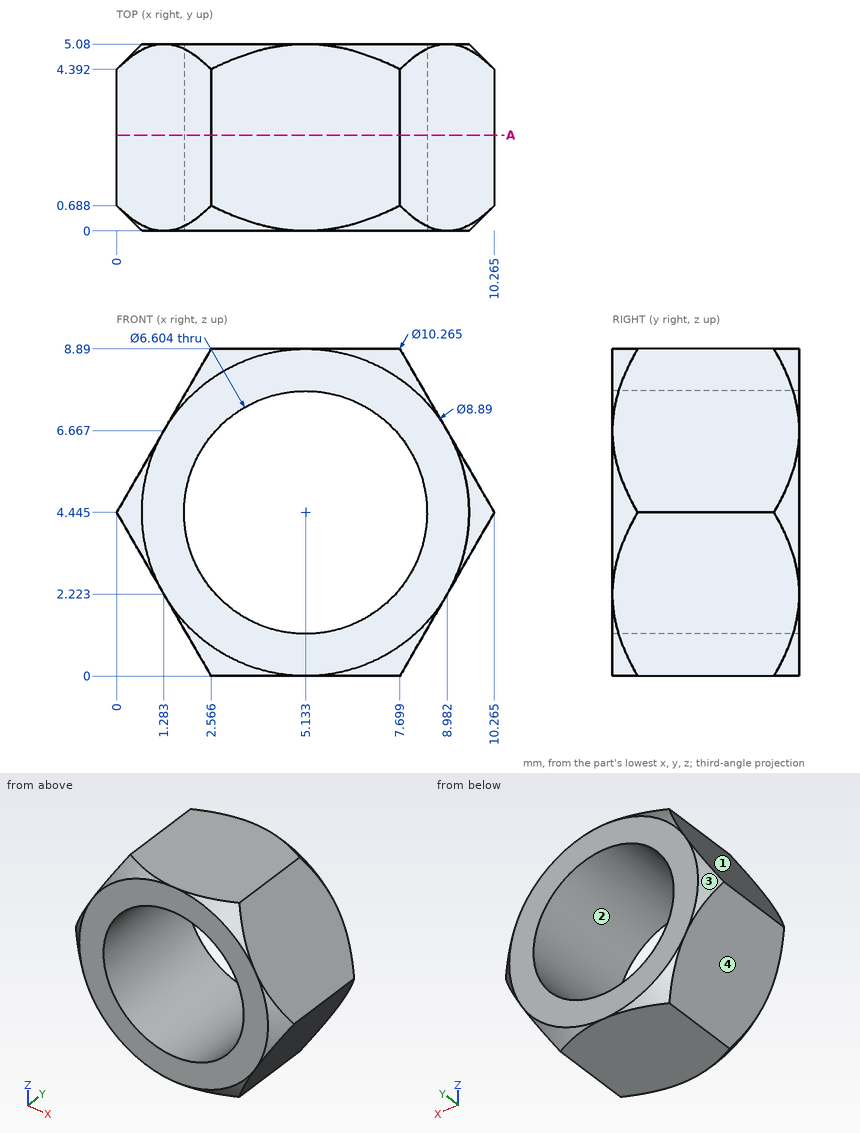
Could you check a few things on this drawing? It's one solid part, dimensions in mm from its lowest x, y, z. Give positions to 0.01 mm unless a question says otherwise; leave off trailing zeros. Order: outer loops, then holes, each group sorted by start corner. A loop starts at its lowest first (then second) coordinate and runs counter-clockwise, first axis right, second up. Notation, with made-up numbers: (32.25, 43) - (78.25, 43) arc R17 cw to (78.25, 76) - close; hole circle Ø7 at (-32, 41.5). An arc over 180 degrees is marked (long way). One line per item, written item: value. Start each with the question number.
1. Imagine slicing it at A-A on y = 2.6. List the corners of the cut face in (x, z) for me (1 decimal).
2. Thinking about a two-plate mould opening in Z: for the marked faces 1, 2, 3 and 4, which applies, +Z half, -Z half, draft (parallel to the pull), parting line (faces both ways), or undercut?
3. If I drill on probe 1 along X at (y, z) = (1.4, 3) (1 decimal); probe 2 along X at (y, z) = (4.4, 6) (1 decimal); probe 3 along Z at (x, y) = (5.25, 4.15) (1 decimal), over which ranges is the centre line in solid material (lowest first)?
4. For P1, Ø3, axis at y = 1.5, z = 2, coming from the +X side, with a flat end and sliding along its axis, tell me the tip position at first contact or that it passes through.
Values:
1. outline: (0, 4.4) - (2.6, 0) - (7.7, 0) - (10.3, 4.4) - (7.7, 8.9) - (2.6, 8.9) - close; hole circle Ø6.6 at (5.1, 4.4)
2. face 1: +Z half
2. face 2: undercut
2. face 3: parting line
2. face 4: -Z half
3. probe 1: 0.8 to 2.2, 8.1 to 9.4
3. probe 2: 0.9 to 2.2, 8 to 9.4
3. probe 3: 0 to 1.1, 7.7 to 8.9
4. P1: x = 9.72
